from build123d import *

# Parameters (mm, degrees)
BOSS_EXTRUDE1_DEPTH = 4.7625


with BuildPart() as part:
    # Sketch1 → Boss-Extrude1 (new body)
    with BuildSketch(Plane.XY):
        Polygon((-26.9875, -101.6), (14.2875, -101.6), (14.2875, -106.3625), (26.9875, -106.3625), (26.9875, -69.85), (31.75, -69.85), (31.75, -38.1), (26.9875, -38.1), (26.9875, -6.35), (31.75, -6.35), (31.75, 25.4), (26.9875, 25.4), (26.9875, 57.15), (31.75, 57.15), (31.75, 88.9), (26.9875, 88.9), (26.9875, 120.65), (31.75, 120.65), (31.75, 152.4), (26.9875, 152.4), (-26.9875, 101.6), align=None)
    extrude(amount=BOSS_EXTRUDE1_DEPTH)


solid = part.part
Check sheet for the modelled part. Datum: model origin and axes. Units: mm. A direction names the side the tool comes from. Round coordinates to 2 decimals unless told otherwise and drop trailing zeros. Write each loop counter-clockwise with the first axis right and the second up, starting at its lowest first coordinate (ties: lowest second). Pieces come first, ordered by that corner, then holes. Notation, with made-up numbers: (16, 59) -> (67, 59) arc R22 cw to (67, 69) -> close; hole circle Ø11 at (50.5, 66). An arc over 180 degrees is marked (long way). Answer as CSV lines item,"result". Start each with the question number.
1) Go/stop test with flat-tipped pins: P1, Ø2.5, axis at x = 30, z = 2.5, coming from the -Y side; P2, Ø1.4, axis at x = -13.5, z = 2.5, coming from the -Y side; P3, Ø2.5, axis at y = 46.5, z = 2, coming from the +X side; P4, Ø4, axis at x = -18.5, y = 0, coming from the -Z side. Record where each tip stops, or that it passes through.
2) Material ranges on line 1 (Y direction, x = 28.5, z = 2.9); line 2 (X direction, y = 37, z = 0.5); line 3 (X direction, y = 132, z = 1.6), recorded low to high. Write a range as from..to.
3) Section check C-C on x = -20. Enter the section's corners in (y, z).
4) Section check A-A on z = 0.9. Enter the section's corners in (x, y).
5) Release check for a two-part mould opening along Y. For faces 4 (the flat face through (26.988, 41, 2)), 5 (the flat face through (-7, -101.6, 2)), 6 (the flat face through (14.288, -104, 2)), 7 (the flat face through (29, 25.4, 2)) record: pulls with the +Y half, pulls with the -Y half, needs draft (parallel to the pull), parting line crosses it, or undercut.
6) Tool access check on faces 1 (the flat face through (26.988, -88, 2)), 2 (the flat face through (31.75, -54, 2)), 3 (the flat face through (29, 57.15, 2)). Record the directions out of +Z, -Z, +X, -X, +Y, -Y that give a thin tool (end or side, any length) a straight path to the whole face; none if there is none.
7) Section check B-B on y = 36. Enter the section's corners in (x, z), and give its area (3 significant figures).
Found:
1,P1,"stops at y = -69.85"
1,P2,"stops at y = -101.6"
1,P3,"stops at x = 26.99"
1,P4,"stops at z = 0"
2,line 1,"y = -69.85..-38.1, -6.35..25.4, 57.15..88.9, 120.65..152.4"
2,line 2,"x = -26.99..26.99"
2,line 3,"x = 5.31..31.75"
3,outline,"(-101.6, 0) -> (108.18, 0) -> (108.18, 4.76) -> (-101.6, 4.76) -> close"
4,outline,"(-26.99, -101.6) -> (14.29, -101.6) -> (14.29, -106.36) -> (26.99, -106.36) -> (26.99, -69.85) -> (31.75, -69.85) -> (31.75, -38.1) -> (26.99, -38.1) -> (26.99, -6.35) -> (31.75, -6.35) -> (31.75, 25.4) -> (26.99, 25.4) -> (26.99, 57.15) -> (31.75, 57.15) -> (31.75, 88.9) -> (26.99, 88.9) -> (26.99, 120.65) -> (31.75, 120.65) -> (31.75, 152.4) -> (26.99, 152.4) -> (-26.99, 101.6) -> close"
5,face 4,"undercut"
5,face 5,"pulls with the -Y half"
5,face 6,"needs draft"
5,face 7,"undercut"
6,face 1,"+Z, -Z, +X, -Y"
6,face 2,"+Z, -Z, +X, +Y, -Y"
6,face 3,"+Z, -Z, +X"
7,outline,"(-26.99, 0) -> (26.99, 0) -> (26.99, 4.76) -> (-26.99, 4.76) -> close"
7,area,"257 mm^2"
